from build123d import *

# Parameters (mm, degrees)
FILLET_R     = 0.2
POCKET_DEPTH = 1.3
FILLET001_R  = 0.2


with BuildPart() as part:
    # Sketch → Revolution (revolve)
    with BuildSketch(Plane.XY):
        Polygon((0, 0), (0, 32), (2.7, 32), (2.7, 30), (1.5, 30), (1.5, 0), align=None)
    revolve(axis=Axis((0, 0, 0), (0, 1, 0)))

    # Fillet
    fillet_edges = [part.edges().sort_by_distance(p)[0] for p in [
        (-2.7, 30, 0),
        (-2.7, 32, 0),
    ]]
    fillet(fillet_edges, radius=FILLET_R)

    # Sketch001 (on Face1 of Fillet) → Pocket (cut)
    with BuildSketch(Plane(origin=(0, 32, 0), x_dir=(-1, 0, 0), z_dir=(0, 1, 0))):
        Polygon((0.5, 1.5), (0.5, 0.5), (1.5, 0.5), (1.5, -0.5), (0.5, -0.5), (0.5, -1.5), (-0.5, -1.5), (-0.5, -0.5), (-1.5, -0.5), (-1.5, 0.5), (-0.5, 0.5), (-0.5, 1.5), align=None)
    extrude(amount=-POCKET_DEPTH, mode=Mode.SUBTRACT)

    # Fillet001
    fillet001_edges = [part.edges().sort_by_distance(p)[0] for p in [
        (0, 32, -1.5),
        (0.5, 32, -1),
        (1, 32, -0.5),
        (1.5, 32, 0),
        (1, 32, 0.5),
        (0.5, 32, 1),
        (-0.5, 32, 1),
        (0, 32, 1.5),
        (-1.5, 32, 0),
        (-1, 32, -0.5),
        (-0.5, 32, -1),
    ]]
    fillet(fillet001_edges, radius=FILLET001_R)


solid = part.part
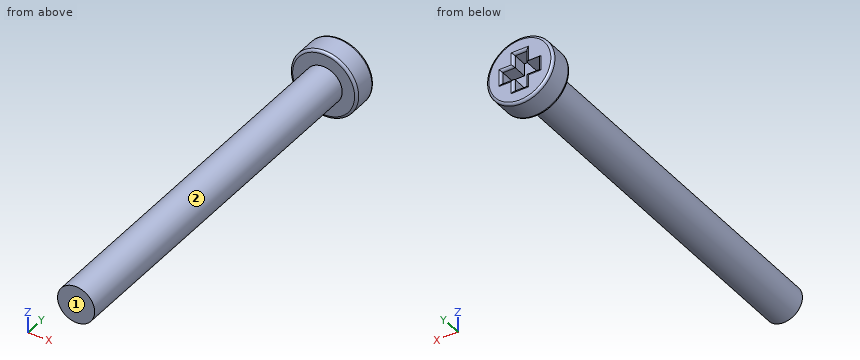
Verification items for the finished model (mm, model axes). Face numbers are marked on the shaded views. A direction names the side the tool comes from. Round coordinates to 2 decimals unless told otherwise and drop trailing zeros. Order: outer loops, then holes, each group sorted by start corner. A loop starts at its lowest first (then second) coordinate and runs counter-clockwise, first axis right, second up.
1. Section check C-C on y = 22.5. Record the cut outline in (x, z), then the cut area to 3 significant figures.
Final values:
outline: circle Ø3 at (0, 0)
area: 7.07 mm2
2. Thickness scan on L1, parallel to Y at x = -1.4, z = -1.6; L2, parallel to Z at x = 0.1, y = 19; L3, parallel to Y at x = -1.4, z = 0.45. Record the ranges inside material, lowest first.
Final values:
L1: y = 30 to 32
L2: z = -1.5 to 1.5
L3: y = 0 to 30.7
3. Section check B-B on z = 0. Record the cut outline in (x, y).
Final values:
outline: (-2.7, 30.2) arc R0.2 ccw to (-2.5, 30) - (-1.5, 30) - (-1.5, 0) - (1.5, 0) - (1.5, 30) - (2.5, 30) arc R0.2 ccw to (2.7, 30.2) - (2.7, 31.8) arc R0.2 ccw to (2.5, 32) - (1.7, 32) arc R0.2 ccw to (1.5, 31.8) - (1.5, 30.7) - (-1.5, 30.7) - (-1.5, 31.8) arc R0.2 ccw to (-1.7, 32) - (-2.5, 32) arc R0.2 ccw to (-2.7, 31.8) - close
4. Go/stop test with flat-tipped pins: P1, Ø1.1, axis at x = -1, y = 31.5, coming from the +Z side; P2, Ø0.5, axis at y = 31, z = 1, coming from the +X side; P3, Ø1, axis at x = 0, y = 12, coming from the -Z side. Record where each tip stops, or that it passes through.
Final values:
P1: stops at z = 2.66
P2: stops at x = 2.59
P3: stops at z = -1.5
5. Section check A-A on x = 0. Record the cut outline in (y, z), then the cut area to 3 significant figures.
Final values:
outline: (0, -1.5) - (30, -1.5) - (30, -2.5) arc R0.2 ccw to (30.2, -2.7) - (31.8, -2.7) arc R0.2 ccw to (32, -2.5) - (32, -1.7) arc R0.2 ccw to (31.8, -1.5) - (30.7, -1.5) - (30.7, 1.5) - (31.8, 1.5) arc R0.2 ccw to (32, 1.7) - (32, 2.5) arc R0.2 ccw to (31.8, 2.7) - (30.2, 2.7) arc R0.2 ccw to (30, 2.5) - (30, 1.5) - (0, 1.5) - close
area: 96.8 mm2
6. Access from +Z, -Z, +X, -X, +Y, -Y to the whole of each face (thin tool, end or side, straight path). Record for the marked faces 1 and 2.
Final values:
face 1: +Z, -Z, +X, -X, -Y
face 2: -Y
